The model under review builds one solid part; all positions refer to its coordinate system, in mm. Round coordinates to 2 decimals unless told otherwise and drop trailing zeros. Loops run counter-clockwise (first coordinate to the right, second up) from the corner with the lowest first, then second, coordinate; pieces in that order, holes last. Notation, with made-up numbers: (52.5, -17) -> (110.5, -17) arc R18 ccw to (110.5, 6) -> close; hole circle Ø5 at (-13, 29). An arc over 180 degrees is marked (long way). Use a Markdown table: item, result. Add a question column.
1) Insertion check: pin 1 (25 mm diameter, centred on x = -119, y = -33.5, fed in from -Z). The pin has a flat end and moves straight along its axis. Give the tip position at first contact, or say it passes through.
2) Consider section B-B on x = -57. Give the boundary of the cut face in (y, z).
3) Consider section C-C on y = 740. Give the boundary of the cut face in (x, z).
4) Consider section A-A on z = 199.5. Give the boundary of the cut face in (x, y).
5) Wall thickness on probe 1 along X at (y, z) = (70, 672); probe 2 along Y at (x, z) = (15.5, 34.5); probe 3 along Z at (x, y) = (-272, 1013): over which ranges is each line inside the solid? List them lowest first.
from build123d import *

# Parameters (mm, degrees)
F1_DEPTH      = 50
F2_W          = 50
F2_H          = 50
F3_DEPTH      = 600
F5_W          = 50
F5_H          = 50
F6_DEPTH      = 500
F6_DEPTH_BACK = 25


with BuildPart() as f1:
    # F0 (on Front) → F1 (new body)
    with BuildSketch(Plane.XZ):
        Polygon((-300, 700), (-300, 0), (300, 0), (300, 700), (250, 700), (250, 50), (-250, 50), (-250, 700), align=None)
    extrude(amount=F1_DEPTH)

    # F4: F3 across plane


with BuildPart() as f3:
    # F2 (on face) → F3 (new body)
    with BuildSketch(Plane(origin=(0, 0, 0), x_dir=(-1, 0, 0), z_dir=(0, 1, 0))):
        with Locations((-275, 675)):
            Rectangle(F2_W, F2_H)
    extrude(amount=F3_DEPTH)


with BuildPart() as f1_1:
    add(f1.part)
    add(f3.part.mirror(Plane.YZ))


    add(f3.part)  # F6 merges F3
    # F5 (on face) → F6 (join, two sides)
    with BuildSketch(Plane.YZ.offset(-250)) as f6_sk:
        with Locations((-25, 675)):
            Rectangle(F5_W, F5_H)
    extrude(amount=F6_DEPTH)
    extrude(f6_sk.sketch, amount=-F6_DEPTH_BACK)

    # F7: F1 across face


with BuildPart() as f1_2:
    add(f1_1.part)
    add(f1_1.part.mirror(Plane(origin=(275, 600, 675), x_dir=(-1, 0, 0), z_dir=(0, 1, 0))))


solid = f1_2.part
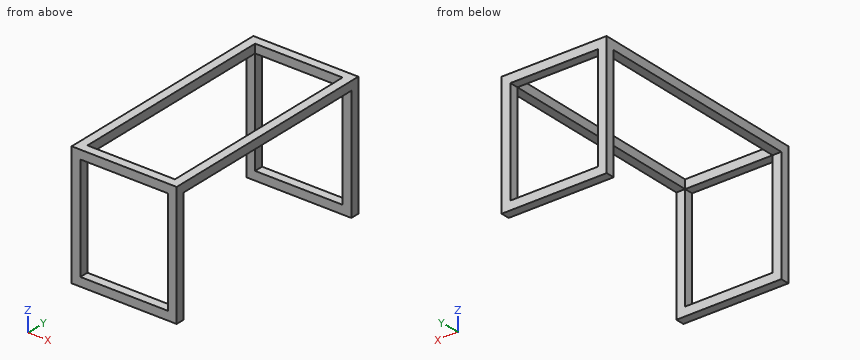
Result set:
| question | item | result |
|---|---|---|
| 1 | pin 1 | z = 0 |
| 2 | outline | (-50, 0) -> (0, 0) -> (0, 50) -> (-50, 50) -> close; (-50, 650) -> (0, 650) -> (0, 700) -> (-50, 700) -> close; (1200, 0) -> (1250, 0) -> (1250, 50) -> (1200, 50) -> close; (1200, 650) -> (1250, 650) -> (1250, 700) -> (1200, 700) -> close |
| 3 | outline | (-300, 650) -> (-250, 650) -> (-250, 700) -> (-300, 700) -> close; (250, 650) -> (300, 650) -> (300, 700) -> (250, 700) -> close |
| 4 | outline | (-300, -50) -> (-250, -50) -> (-250, 0) -> (-300, 0) -> close; (-300, 1200) -> (-250, 1200) -> (-250, 1250) -> (-300, 1250) -> close; (250, -50) -> (300, -50) -> (300, 0) -> (250, 0) -> close; (250, 1200) -> (300, 1200) -> (300, 1250) -> (250, 1250) -> close |
| 5 | probe 1 | -300 to -250, 250 to 300 |
| 5 | probe 2 | -50 to 0, 1200 to 1250 |
| 5 | probe 3 | 650 to 700 |
